Design review of the part shown in the three views and the two pictorial views. Dimensions are in mm from the part's minimum x, y and z. A direction names the side the tool comes from. Round coordinates to 2 decimals unless told otherwise and drop trailing zeros. Loops run counter-clockwise (first coordinate to the right, second up) from the corner with the lowest first, then second, coordinate; pieces in that order, holes last. Notation, with made-up numbers: M 46,-36 L 56,-36 A23 cw 56,-1 Z; hole C 51.25,-23.75 d4. An arc over 180 degrees is marked long. Return JSON: item names as keys, results as strings. Group by question number.
Q1. To check wall thickness, follow line 1 along X through (y, z) = (30, 23); line 2 along X through (y, z) = (52, 7); line 3 along Y through (x, z) = (53, 21.5). State the ranges of each line that lie inside material, in increasing order.
Q2. Clearance check with flat-ended pins moving along their axes: pin 1 Ø12 at (y, z) = (82.5, 22) entering from +X; pin 2 Ø6 at (y, z) = (58, 5.5) entering from -X; pin 3 Ø6 at (x, z) = (67.5, 40) entering from +Y. State where each tip first meets the part, or that it passes through.
Q3. Consider section C-C (z = 25.5). State the section outline as (x, y) points.
Q4. Draft analysis for pull direction X (two halves, no side actions). For the marked faces 3, 4 and 5, state which applies: pulls with the +X half, pulls with the -X half, needs draft (parallel to the pull), parting line crosses it, or undercut.
Q5. Consider section D-D (z = 5.5). State the section outline as (x, y) points, and give its area (3 significant figures).
Q6. Consider section A-A (y = 53). State the section outline as (x, z) points.
Q7. For the marked faces 1 and 2, list the 3-axis set-ups (+Z, -Z, +X, -X, +Y, -Y) from which the entire face can be reached by the end or side of a thin tool; tool diameter is ignored.
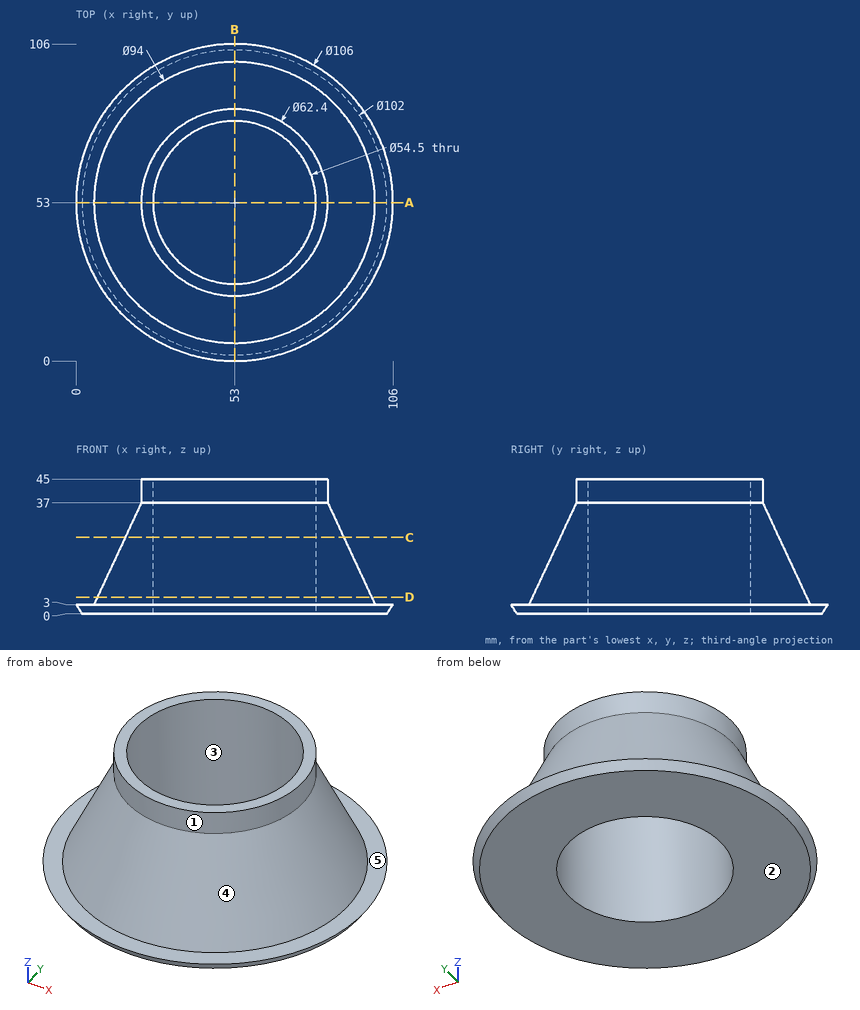
Values:
{
 "1": {"line 1": "x = 23.12 to 38.39, 67.61 to 82.88", "line 2": "x = 7.87 to 25.77, 80.23 to 98.13", "line 3": "y = 14.6 to 25.75, 80.25 to 91.4"},
 "2": {"pin 1": "stops at x = 84.26", "pin 2": "stops at x = 0.11", "pin 3": "stops at y = 82"},
 "3": {"outline": "C 53,53 d73.09; hole C 53,53 d54.5"},
 "4": {"face 3": "undercut", "face 4": "parting line crosses it", "face 5": "needs draft"},
 "5": {"outline": "C 53,53 d91.68; hole C 53,53 d54.5", "area": "4,270 mm2"},
 "6": {"outline": "M 0,3 L 2,0 L 25.75,0 L 25.75,45 L 21.8,45 L 21.8,37 L 6,3 Z; M 80.25,0 L 104,0 L 106,3 L 100,3 L 84.2,37 L 84.2,45 L 80.25,45 Z"},
 "7": {"face 1": "+Z", "face 2": "-Z, +X, -X, +Y, -Y"}
}
